Source: CAD feature listing. Evaluate the final solid. Frame: model axes, mm. Face numbers are marked on the shaded views. A direction names the side the tool comes from. Give positions to 0.01 mm unless a question says otherwise; leave off trailing zeros. Write each loop counter-clockwise with the first axis right and the second up, starting at its lowest first coordinate (ties: lowest second). Pieces come first, ordered by that corner, then holes. Notation, with made-up numbers: (30, 68.5) -> (87, 68.5) arc R17 cw to (87, 92.5) -> close; hole circle Ø5 at (30, 70). An arc over 180 degrees is marked (long way). Answer as a JSON object with one key per item and string values. Group by question number.
Item 1: Section query D-D on y = -15.5. Return the cut outline in (x, z), plus the area to 3 significant figures.
Item 2: Section query A-A on z = 24.5. Return the cut outline in (x, y), plus the area to 3 significant figures.
Item 3: Section query B-B on x = -3.5. Return the cut outline in (y, z).
Item 4: First-contact query: pin 1 Ø12 at (y, z) = (0, 41.5) entering from -X; pin 2 Ø2.5 at (x, y) = (16, 15) entering from +Z; pin 3 Ø0.9 at (x, y) = (-16, 15.5) entering from +Z. Flat tips, straight axial feed; report the tip coordinate or a pass-through.
Item 5: Ray query, probe 1 along X at (y, z) = (-15, 28); probe 2 along Z at (x, y) = (-2.5, 17.5); probe 3 along Z at (x, y) = (6, 3). Return the intervals inside material, ascending. Write a range as from..to.
Item 6: Section query C-C on y = 0. Return the cut outline in (x, z).
Item 7: Access query for the marked faces 1 and 2. Directions: +Z, -Z, +X, -X, +Y, -Y. A direction counts if a zero-diameter tool reaches every point of the face in a straight line with its end or side. Return the directions, or none.
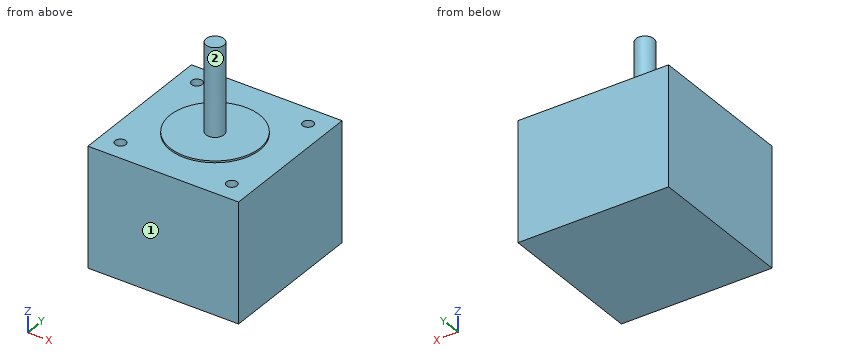
from build123d import *

# Parameters (mm, degrees)
SKETCH_1_W          = 42
SKETCH_1_H          = 42
EXTRUDE_1_DEPTH     = 33.3
SKETCH_2_R          = 12.5
EXTRUDE_2_DEPTH     = 0.5
SKETCH_3_R          = 1.5
CUT_EXTRUDE_1_DEPTH = 10
SKETCH_5_R          = 2.5
EXTRUDE_3_DEPTH     = 25


with BuildPart() as part:
    # ｽｹｯﾁ1 → ﾎﾞｽ - 押し出し1 (new body)
    with BuildSketch(Plane.XY):
        Rectangle(SKETCH_1_W, SKETCH_1_H)
    extrude(amount=EXTRUDE_1_DEPTH)

    # ｽｹｯﾁ2 → ﾎﾞｽ - 押し出し2 (add)
    with BuildSketch(Plane.XY.offset(33.3)):
        Circle(SKETCH_2_R)
    extrude(amount=EXTRUDE_2_DEPTH)

    # ｽｹｯﾁ3 → ｶｯﾄ - 押し出し1 (cut)
    with BuildSketch(Plane.XY.offset(33.3)):
        with Locations((-15.682538541, 15.5)):
            Circle(SKETCH_3_R)
        with Locations((-15.682538541, -15.5)):
            Circle(SKETCH_3_R)
        with Locations((15.317461459, -15.5)):
            Circle(SKETCH_3_R)
        with Locations((15.317461459, 15.5)):
            Circle(SKETCH_3_R)
    extrude(amount=-CUT_EXTRUDE_1_DEPTH, mode=Mode.SUBTRACT)

    # ｽｹｯﾁ5 → ﾎﾞｽ - 押し出し3 (add)
    with BuildSketch(Plane.XY.offset(33.3)):
        Circle(SKETCH_5_R)
    extrude(amount=EXTRUDE_3_DEPTH)


solid = part.part
Worked answers:
{
 "1": {"outline": "(-21, 0) -> (21, 0) -> (21, 33.3) -> (16.82, 33.3) -> (16.82, 23.3) -> (13.82, 23.3) -> (13.82, 33.3) -> (-14.18, 33.3) -> (-14.18, 23.3) -> (-17.18, 23.3) -> (-17.18, 33.3) -> (-21, 33.3) -> close", "area": "1,340 mm^2"},
 "2": {"outline": "(-21, -21) -> (21, -21) -> (21, 21) -> (-21, 21) -> close; hole circle Ø3 at (-15.68, -15.5); hole circle Ø3 at (-15.68, 15.5); hole circle Ø3 at (15.32, -15.5); hole circle Ø3 at (15.32, 15.5)", "area": "1,740 mm^2"},
 "3": {"outline": "(-21, 0) -> (21, 0) -> (21, 33.3) -> (12, 33.3) -> (12, 33.8) -> (-12, 33.8) -> (-12, 33.3) -> (-21, 33.3) -> close"},
 "4": {"pin 1": "x = -2.5", "pin 2": "z = 33.3", "pin 3": "z = 23.3"},
 "5": {"probe 1": "-21..-17.1, -14.27..13.9, 16.73..21", "probe 2": "0..33.3", "probe 3": "0..33.8"},
 "6": {"outline": "(-21, 0) -> (21, 0) -> (21, 33.3) -> (12.5, 33.3) -> (12.5, 33.8) -> (2.5, 33.8) -> (2.5, 58.3) -> (-2.5, 58.3) -> (-2.5, 33.8) -> (-12.5, 33.8) -> (-12.5, 33.3) -> (-21, 33.3) -> close"},
 "7": {"face 1": "+Z, -Z, +X, -X, -Y", "face 2": "+Z"}
}
